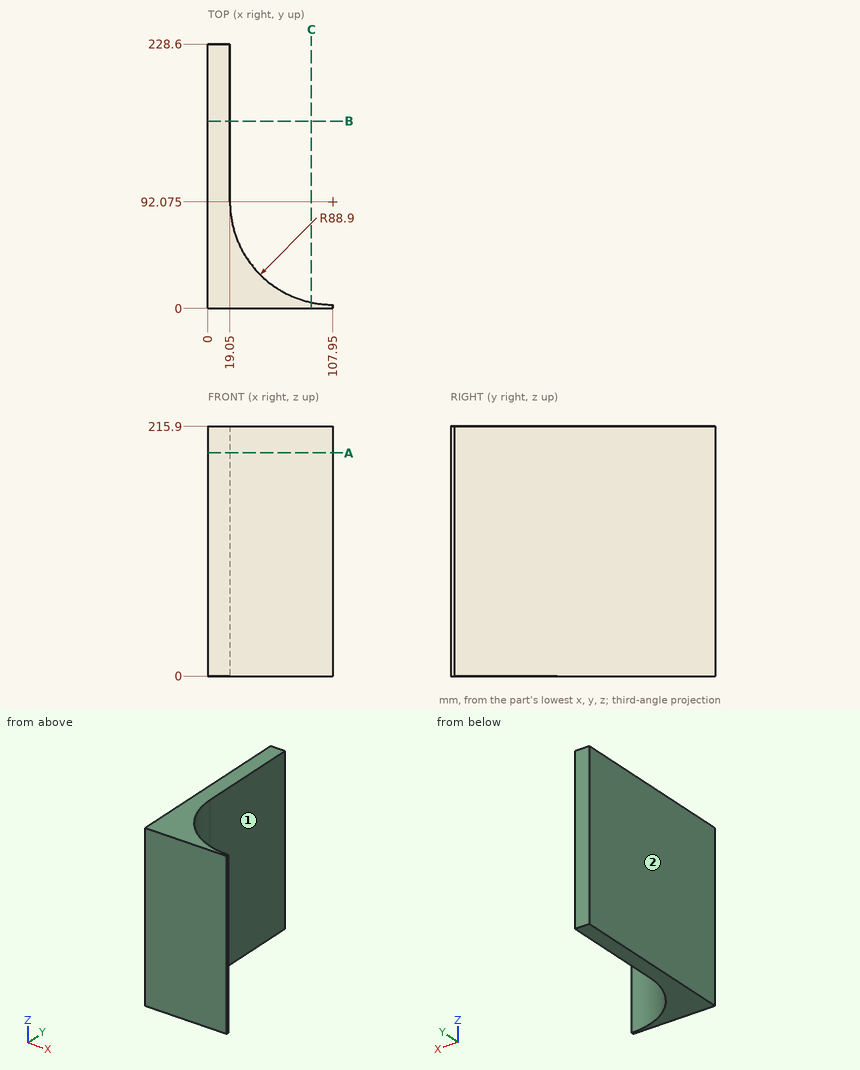
Part print with two shaded views. Sizes in mm from the minimum x, y, z corner. A direction names the side the tool comes from. Coordinates: 2 decimals unless noted, no trailing zeros. Write each loop counter-clockwise with the first axis right and the second up, starting at its lowest first coordinate (ties: lowest second). Pieces come first, ordered by that corner, then holes. Notation, with made-up numbers: (-13.5, -33) - (6.5, -33) arc R11 cw to (6.5, -22) - close; hole circle Ø8 at (0.5, 12.5). An arc over 180 degrees is marked (long way). One line per item, written item: value. Start each with the question number.
1. Tool access for the marked faces 1 and 2: list every direction of +Z, -Z, +X, -X, +Y, -Y with a clear straight run to the whole face (end or side of a thin tool).
2. Flat gauge pins, fed straight in: pin 1 (5 mm diameter, centred on x = 75.5, z = 153.5, fed in from -Y); pin 2 (12 mm diameter, centred on x = 62, z = 100, fed in from +Y); pin 3 (5 mm diameter, centred on y = 50.5, z = 23.5, fed in from +X). Where does each tip first touch, or does it go through?
3. Probe line 1 (X direction, y = 89, z = 45); line 2 (Y direction, x = 80, z = 178); line 3 (Y direction, x = 100, z = 29.5). List the from-to ranges inside material, lowest first. Write a range as from..to.
4. Slice it at A-A (z = 193). Write the cut outline in (x, y) (3 decimals).
5. Slice it at B-B (y = 162). Write the cut outline in (x, z).
6. Slice it at C-C (x = 89.5). Write the cut outline in (y, z), plus the area to 3 significant figures.
Answers below:
1. face 1: +Z, -Z, +X, +Y
1. face 2: +Z, -Z, -X, +Y, -Y
2. pin 1: stops at y = 0
2. pin 2: stops at y = 19.93
2. pin 3: stops at x = 30.75
3. line 1: x = 0..19.1
3. line 2: y = 0..7.68
3. line 3: y = 0..3.53
4. outline: (0, 0) - (107.95, 0) - (107.95, 3.175) arc R88.9 cw to (19.05, 92.075) - (19.05, 228.6) - (0, 228.6) - close
5. outline: (0, 0) - (19.05, 0) - (19.05, 215.9) - (0, 215.9) - close
6. outline: (0, 0) - (5.11, 0) - (5.11, 215.9) - (0, 215.9) - close
6. area: 1,100 mm^2
